```python
from build123d import *

# Parameters (mm, degrees)
SKETCH_1_R               = 22
SKETCH_1_R_2             = 12
EXTRUDE_1_DEPTH          = 5
SKETCH_1_3_R             = 2.7
CUT_EXTRUDE_1_DEPTH      = 32.511902513
PATTERN_CIRCULAR_1_COUNT = 3


with BuildPart() as part:
    # Sketch 1 → Extrude 1 (new body)
    with BuildSketch(Plane(origin=(0, 0, 0), x_dir=(1, 0, 0), z_dir=(0, 1, 0))):
        with Locations(Location((0, 0, 0), (0, 0, 270))):
            Circle(SKETCH_1_R)
        with Locations(Location((0, 0, 0), (0, 0, 270))):
            Circle(SKETCH_1_R_2, mode=Mode.SUBTRACT)
    extrude(amount=EXTRUDE_1_DEPTH)

    # Sketch 1_3 → Cut-Extrude 1 (cut, symmetric)
    with BuildSketch(Plane(origin=(0, 0, 0), x_dir=(1, 0, 0), z_dir=(0, 1, 0))):
        with Locations(Location((0, 17.5, 0), (0, 0, 270))):
            Circle(SKETCH_1_3_R)
    cut_extrude_1 = extrude(amount=CUT_EXTRUDE_1_DEPTH, both=True, mode=Mode.SUBTRACT)

    # Pattern Circular 1: Cut-Extrude 1 ×3 about axis
    pattern_circular_1_axis = Axis((0, 0, 0), (0, 1, 0))
    for i in range(1, PATTERN_CIRCULAR_1_COUNT):
        add(cut_extrude_1.rotate(pattern_circular_1_axis, i * 360 / PATTERN_CIRCULAR_1_COUNT), mode=Mode.SUBTRACT)


solid = part.part
```
Geometry check sheet. Reference: the model listing, model coordinates, mm. Give positions to 0.01 mm unless a question says otherwise; leave off trailing zeros. Order: outer loops, then holes, each group sorted by start corner. A loop starts at its lowest first (then second) coordinate and runs counter-clockwise, first axis right, second up. Notation, with made-up numbers: (3, 62.5) - (58, 62.5) arc R14 cw to (58, 67.5) - close; hole circle Ø1 at (42, 62.5). An arc over 180 degrees is marked (long way). Write item = value, one per line. Start each with the question number.
1) Section check C-C (x = -10.5). Enter the section's corners in (y, z), then the cut area to 3 significant figures.
2) Draft check along Z on faces 1 (the cylindrical face through (3.604, 2.465, 11.446)), 2 (the flat face through (-9, 0, 9)), 3 (the cylindrical face through (15.966, 2.535, 11.325)), 4 (the cylindrical face through (-21.477, 2.465, -4.769)). Enter one of: released by +Z, released by -Z, zero draft, split by the parting line, or undercut.
3) Section check A-A (x = 0). Enter the section's corners in (y, z), then the cut area to 3 significant figures.
4) Scan lines: L1, parallel to X at y = 1.45, z = 8.75; L2, parallel to X at y = 2.5, z = -0.5; L3, parallel to Z at x = 10.5, y = 2.45. Record each from-to range of solid material in increasing order.
5) Section check B-B (z = 5.5). Enter the section's corners in (x, y), then the cut area to 3 significant figures.
6) Section check D-D (z = 10.5). Enter the section's corners in (x, y).
7) Gauge pin test, flat ends, axial feed: pin 1 Ø6 at (x, z) = (15.16, 8.75) entering from +Y; pin 2 Ø3 at (y, z) = (4.5, 5) entering from +X; pin 3 Ø3 at (y, z) = (2.5, 1) entering from +X. Record the tip position at first contact, or that the pin passes through.
Geometry check:
q1.outline = (0, -19.33) - (5, -19.33) - (5, -5.81) - (0, -5.81) - close; (0, 5.81) - (5, 5.81) - (5, 19.33) - (0, 19.33) - close
q1.area = 135 mm2
q2.face_1 = undercut
q2.face_2 = zero draft
q2.face_3 = undercut
q2.face_4 = split by the parting line
q3.outline = (0, -22) - (5, -22) - (5, -20.2) - (0, -20.2) - close; (0, -14.8) - (5, -14.8) - (5, -12) - (0, -12) - close; (0, 12) - (5, 12) - (5, 22) - (0, 22) - close
q3.area = 73.0 mm2
q4.L1 = -20.19 to -17.86, -12.46 to -8.21, 8.21 to 12.46, 17.86 to 20.19
q4.L2 = -21.99 to -11.99, 11.99 to 21.99
q4.L3 = -19.33 to -5.81, 5.81 to 19.33
q5.outline = (-21.3, 0) - (-10.67, 0) - (-10.67, 5) - (-21.3, 5) - close; (10.67, 0) - (21.3, 0) - (21.3, 5) - (10.67, 5) - close
q5.area = 106 mm2
q6.outline = (-19.33, 0) - (-17.21, 0) - (-17.21, 5) - (-19.33, 5) - close; (-13.1, 0) - (-5.81, 0) - (-5.81, 5) - (-13.1, 5) - close; (5.81, 0) - (13.1, 0) - (13.1, 5) - (5.81, 5) - close; (17.21, 0) - (19.33, 0) - (19.33, 5) - (17.21, 5) - close
q7.pin_1 = 5
q7.pin_2 = 21.72
q7.pin_3 = 22
